Check sheet for the modelled part. Datum: model origin and axes. Units: mm. A direction names the side the tool comes from. Give positions to 0.01 mm unless a question says otherwise; leave off trailing zeros. Order: outer loops, then holes, each group sorted by start corner. A loop starts at its lowest first (then second) coordinate and runs counter-clockwise, first axis right, second up.
Item 1: Access from +Z, -Z, +X, -X, +Y, -Y to the whole of each face (thin tool, end or side, straight path). Record for faces 1 (the flat face through (15, 22, 41.825)), 2 (the cylindrical face through (19.672, 12.335, 43.435)).
Item 2: Gauge pin test, flat ends, axial feed: P1, Ø5, axis at x = 6, y = 15, coming from the -Z side (3 decimals); P2, Ø19, axis at x = 22.5, z = 22, coming from the +Y side (3 decimals). Record the tip position at first contact, or that the pin passes through.
Item 3: Sectioned sample at D-D on y = 27. Record the boundary of the cut face in (x, z) (3 decimals), and give its area (3 significant figures).
Item 4: Release check for a two-part mould opening along X. For faces 3 (the flat face through (19, 0, 22)), 4 (the cylindrical face through (19.58, 32.06, 43.43)), 5 (the flat face through (0, 2, 33)) record: released by +X, released by -X, zero draft, split by the parting line, or undercut.
Item 5: Sectioned sample at C-C on x = 19. Record the boundary of the cut face in (y, z) (3 decimals), and give its area (3 significant figures).
Item 6: Sectioned sample at B-B on z = 4. Record the boundary of the cut face in (x, y) (3 decimals), and give its area (3 significant figures).
Item 7: Sectioned sample at A-A on x = 4. Record the boundary of the cut face in (y, z) (3 decimals).
Item 8: Material ranges on line 1 along Y through (x, z) = (19, 43) (3 decimals); line 2 along Z through (x, y) = (16, 14) (3 decimals); line 3 along Y through (x, z) = (33, 18) (3 decimals), recorded low to high.
from build123d import *

# Parameters (mm, degrees)
SKETCH1_W            = 38
SKETCH1_H            = 45
BOSS_EXTRUDE1_DEPTH  = 3.175
SKETCH2_W            = 38
SKETCH2_H            = 3.175
BOSS_EXTRUDE2_DEPTH  = 38.1
SKETCH3_R            = 1.25
CAMERA_HOLES_DEPTH   = 10
SKETCH4_R            = 1.25
MOUNTING_HOLES_DEPTH = 10


with BuildPart() as part:
    # Sketch1 → Boss-Extrude1 (new body)
    with BuildSketch(Plane(origin=(0, 0, 0), x_dir=(1, 0, 0), z_dir=(0, 1, 0))):
        with Locations((19, -22.5)):
            Rectangle(SKETCH1_W, SKETCH1_H)
    extrude(amount=BOSS_EXTRUDE1_DEPTH)

    # Sketch2 → Boss-Extrude2 (add)
    with BuildSketch(Plane(origin=(0, 3.175, 0), x_dir=(1, 0, 0), z_dir=(0, 1, 0))):
        with Locations((19, -43.4125)):
            Rectangle(SKETCH2_W, SKETCH2_H)
    extrude(amount=BOSS_EXTRUDE2_DEPTH)

    # Sketch3 → camera holes (cut)
    with BuildSketch(Plane.XZ):
        with Locations((4, 34)):
            Circle(SKETCH3_R)
        with Locations((34, 34)):
            Circle(SKETCH3_R)
        with Locations((4, 4)):
            Circle(SKETCH3_R)
        with Locations((34, 4)):
            Circle(SKETCH3_R)
    extrude(amount=-CAMERA_HOLES_DEPTH, mode=Mode.SUBTRACT)

    # Sketch4 → mounting holes (cut)
    with BuildSketch(Plane.XY.offset(45)):
        with Locations((19, 11.28125)):
            Circle(SKETCH4_R)
        with Locations((19, 33.16875)):
            Circle(SKETCH4_R)
        with Locations((19, 22.225)):
            Circle(SKETCH4_R)
    extrude(amount=-MOUNTING_HOLES_DEPTH, mode=Mode.SUBTRACT)


solid = part.part
Report:
1. face 1: -Z, +X, -X, +Y
1. face 2: +Z, -Z
2. P1: stops at z = 41.825
2. P2: stops at y = 3.175
3. outline: (0, 41.825) - (38, 41.825) - (38, 45) - (0, 45) - close
3. area: 121 mm2
4. face 3: zero draft
4. face 4: undercut
4. face 5: released by -X
5. outline: (0, 0) - (3.175, 0) - (3.175, 41.825) - (10.031, 41.825) - (10.031, 45) - (0, 45) - close; (12.531, 41.825) - (20.975, 41.825) - (20.975, 45) - (12.531, 45) - close; (23.475, 41.825) - (31.919, 41.825) - (31.919, 45) - (23.475, 45) - close; (34.419, 41.825) - (41.275, 41.825) - (41.275, 45) - (34.419, 45) - close
5. area: 240 mm2
6. outline: (0, 0) - (2.75, 0) - (2.75, 3.175) - (0, 3.175) - close; (5.25, 0) - (32.75, 0) - (32.75, 3.175) - (5.25, 3.175) - close; (35.25, 0) - (38, 0) - (38, 3.175) - (35.25, 3.175) - close
6. area: 105 mm2
7. outline: (0, 0) - (3.175, 0) - (3.175, 2.75) - (0, 2.75) - close; (0, 5.25) - (3.175, 5.25) - (3.175, 32.75) - (0, 32.75) - close; (0, 35.25) - (3.175, 35.25) - (3.175, 41.825) - (41.275, 41.825) - (41.275, 45) - (0, 45) - close
8. line 1: y = 0 to 10.031, 12.531 to 20.975, 23.475 to 31.919, 34.419 to 41.275
8. line 2: z = 41.825 to 45
8. line 3: y = 0 to 3.175
